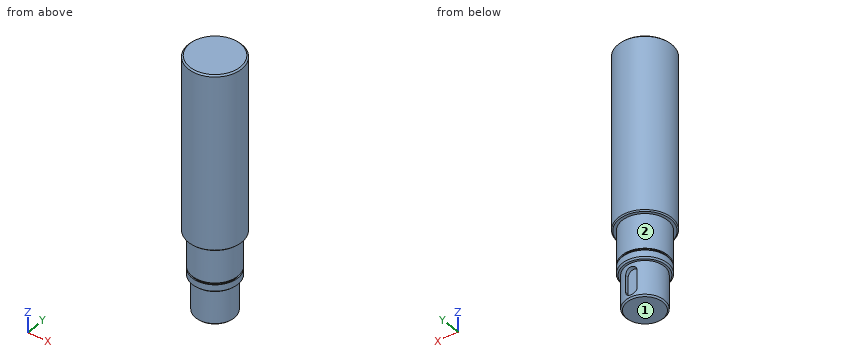
from build123d import *

# Parameters (mm, degrees)
CHAMFER_1_SIZE      = 2
CHAMFER_2_SIZE      = 1.5
CUT_EXTRUDE_1_DEPTH = 6
CHAMFER_3_SIZE      = 2


with BuildPart() as part:
    # Эскиз1 → Повернуть1 (revolve)
    with BuildSketch(Plane(origin=(0, 0, 0), x_dir=(0, 0, -1), z_dir=(1, 0, 0)), mode=Mode.PRIVATE) as revolve_1_sk:
        Polygon((0, 0), (0, 38), (250, 38), (250, 32.5), (299.35, 32.5), (299.35, 31), (302, 31), (302, 32.5), (313, 32.5), (313, 27.5), (363, 27.5), (363, 0), align=None)
    revolve(revolve_1_sk.sketch.rotate(Axis((0, 0, 0), (0, 0, -1)), 90), axis=Axis((0, 0, 0), (0, 0, -1)))

    # Фаска1
    chamfer_1_edges = [part.edges().sort_by_distance(p)[0] for p in [
        (-38, 0, 0),
        (-27.5, 0, -363),
    ]]
    chamfer(chamfer_1_edges, length=CHAMFER_1_SIZE)

    # Фаска2
    chamfer_2_edges = [part.edges().sort_by_distance(p)[0] for p in [
        (-38, 0, -250),
    ]]
    chamfer(chamfer_2_edges, length=CHAMFER_2_SIZE)

    # Эскиз8 → Вырез-Вытянуть1 (cut)
    with BuildSketch(Plane(origin=(-6.6, 27.5, -280), x_dir=(-1, 0, 0), z_dir=(0, -1, 0))):
        with BuildLine():
            Line((1.4, 70), (1.4, 46))
            ThreePointArc((1.4, 46), (-6.6, 38), (-14.6, 46))
            Line((-14.6, 46), (-14.6, 70))
            ThreePointArc((-14.6, 70), (-6.6, 78), (1.4, 70))
        make_face()
    extrude(amount=CUT_EXTRUDE_1_DEPTH, mode=Mode.SUBTRACT)

    # Фаска3
    chamfer_3_edges = [part.edges().sort_by_distance(p)[0] for p in [
        (-32.5, 0, -313),
    ]]
    chamfer(chamfer_3_edges, length=CHAMFER_3_SIZE)


solid = part.part
Input: part model. Units: mm. Frame: model coordinates. Face numbers are marked on the shaded views. A direction names the side the tool comes from. Coordinates: 2 decimals unless noted, no trailing zeros. Loops run counter-clockwise (first coordinate to the right, second up) from the corner with the lowest first, then second, coordinate; pieces in that order, holes last.
Q1. Set-up query: the marked faces 1 and 2. Return all of +Z, -Z, +X, -X, +Y, -Y with unobstructed straight access to the full face (end or side cutting, diameter ignored); none if empty.
Q2. Cut plane C-C (z = -37.5). Output: boundary loops of the cut face in (x, y).
Q3. Cut plane D-D (z = -338). Output: boundary loops of the cut face in (x, y).
Q4. Material intervals for line 1 (X direction, y = -2, z = -96); line 2 (Y direction, x = 1, z = -344); line 3 (Z direction, x = 20.5, y = 27), sorted ascending.
Q5. Contact query for flat-ended pins moving along their axis: pin 1 (8 mm diameter, centred on x = -5, z = -199, fed in from +Y); pin 2 (5 mm diameter, centred on x = 2, z = -338, fed in from +Y); pin 3 (12 mm diameter, centred on y = -20.5, z = -237, fed in from -X). Output: stop coordinate, or through.
Q6. Cut plane A-A (y = 0). Output: boundary loops of the cut face in (x, z), then the cut area to 3 significant figures.
Working result:
1. face 1: -Z, +X, -X, +Y, -Y
1. face 2: -Z
2. outline: circle Ø76 at (0, 0)
3. outline: (-8, 21.5) - (-8, 26.31) arc R27.5 ccw (long way) to (8, 26.31) - (8, 21.5) - close
4. line 1: x = -37.95 to 37.95
4. line 2: y = -27.48 to 21.5
4. line 3: z = -250 to 0
5. pin 1: stops at y = 37.99
5. pin 2: stops at y = 21.5
5. pin 3: stops at x = -35.12
6. outline: (-38, -248.5) - (-36.5, -250) - (-32.5, -250) - (-32.5, -299.35) - (-31, -299.35) - (-31, -302) - (-32.5, -302) - (-32.5, -311) - (-30.5, -313) - (-27.5, -313) - (-27.5, -361) - (-25.5, -363) - (25.5, -363) - (27.5, -361) - (27.5, -313) - (30.5, -313) - (32.5, -311) - (32.5, -302) - (31, -302) - (31, -299.35) - (32.5, -299.35) - (32.5, -250) - (36.5, -250) - (38, -248.5) - (38, -2) - (36, 0) - (-36, 0) - (-38, -2) - close
6. area: 25,800 mm2
